Design review of the part built by this model. Coordinates are the model's own, in mm. Face numbers are marked on the shaded views. A direction names the side the tool comes from. Give positions to 0.01 mm unless a question says otherwise; leave off trailing zeros. Order: outer loops, then holes, each group sorted by start corner. A loop starts at its lowest first (then second) coordinate and runs counter-clockwise, first axis right, second up. Notation, with made-up numbers: (-24, 19) -> (27, 19) arc R23 cw to (27, 31) -> close; hole circle Ø6 at (68, -11.5). An arc over 180 degrees is marked (long way). One line per item, written item: value.
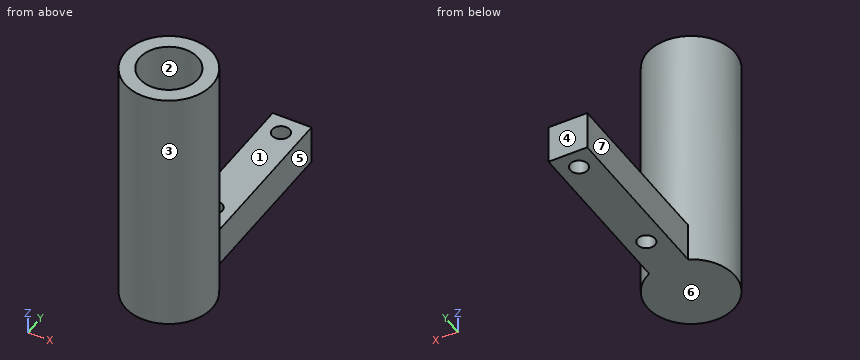
from build123d import *

# Parameters (mm, degrees)
ESQUISSE1_R             = 22.5
BASE_EXTRUSION_DEPTH    = 130
ESQUISSE2_W             = 20
ESQUISSE2_H             = 20
BOSS_EXTRU_1_DEPTH      = 110
ESQUISSE3_R             = 4.5
ENL_V_MAT_EXTRU_1_DEPTH = 20
ESQUISSE4_R             = 15
ENL_V_MAT_EXTRU_2_DEPTH = 120


with BuildPart() as part:
    # Esquisse1 → Base-Extrusion (new body)
    with BuildSketch(Plane.XY):
        with Locations(Location((0, 0, 0), (0, 0, 116.387799961))):
            Circle(ESQUISSE1_R)
    extrude(amount=BASE_EXTRUSION_DEPTH)

    # Esquisse2 → Boss.-Extru.1 (add)
    with BuildSketch(Plane(origin=(0, 0, 0), x_dir=(1, 0, 0), z_dir=(0, 1, 0))):
        with Locations((0, -10)):
            Rectangle(ESQUISSE2_W, ESQUISSE2_H)
    extrude(amount=BOSS_EXTRU_1_DEPTH)

    # Esquisse3 → Enlèv. mat.-Extru.1 (cut)
    with BuildSketch(Plane.XY.offset(20)):
        with Locations((0, 100)):
            Circle(ESQUISSE3_R)
        with Locations((0, 40)):
            Circle(ESQUISSE3_R)
    extrude(amount=-ENL_V_MAT_EXTRU_1_DEPTH, mode=Mode.SUBTRACT)

    # Esquisse4 → Enlèv. mat.-Extru.2 (cut)
    with BuildSketch(Plane.XY.offset(130)):
        Circle(ESQUISSE4_R)
    extrude(amount=-ENL_V_MAT_EXTRU_2_DEPTH, mode=Mode.SUBTRACT)


solid = part.part
Item 1: Machinability: for the marked faces 5, 6 and 7, which of the approach directions +Z, -Z, +X, -X, +Y, -Y give a long, thin tool a straight path to every point of the face, cutting with its end or side? Answer none if there is none.
Returned:
face 5: +Z, -Z, +X, +Y
face 6: -Z, +X, -X, +Y, -Y
face 7: +Z, -Z, -X, +Y
Item 2: Clearance check with flat-ended pins moving along their axes: P1, Ø10, axis at x = -17.5, z = 57.5, coming from the -Y side; P2, Ø3, axis at x = 7.5, z = 92, coming from the -Y side; P3, Ø6, axis at x = 7.5, z = 85, coming from the -Y side; P4, Ø8, axis at x = 0, y = 100, coming from the -Z side. State where each tip first meets the part, or that it passes through.
Returned:
P1: y = -18.71
P2: y = -21.69
P3: y = -22.05
P4: through
Item 3: Add section D-D on y = 0. Give the boundary of the cut face in (x, z).
Returned:
outline: (-22.5, 0) -> (22.5, 0) -> (22.5, 130) -> (15, 130) -> (15, 10) -> (-15, 10) -> (-15, 130) -> (-22.5, 130) -> close
Item 4: Add section C-C on z = 14. Give the boundary of the cut face in (x, y).
Returned:
outline: (-10, 20.16) arc R22.5 ccw (long way) to (10, 20.16) -> (10, 110) -> (-10, 110) -> close; hole circle Ø30 at (0, 0); hole circle Ø9 at (0, 40); hole circle Ø9 at (0, 100)
Item 5: To check wall thickness, follow line 1 along Y through (x, z) = (0, 13); line 2 along Y through (x, z) = (0, 9); line 3 along Y through (x, z) = (0, 69). State the ranges of each line that lie inside material, in increasing order. Write a range as from..to.
Returned:
line 1: -22.5..-15, 15..35.5, 44.5..95.5, 104.5..110
line 2: -22.5..35.5, 44.5..95.5, 104.5..110
line 3: -22.5..-15, 15..22.5
Item 6: Add section A-A on y = 100. Give the boundary of the cut face in (x, z).
Returned:
outline: (-10, 0) -> (-4.5, 0) -> (-4.5, 20) -> (-10, 20) -> close; (4.5, 0) -> (10, 0) -> (10, 20) -> (4.5, 20) -> close
Item 7: Add section B-B on x = 0.5. Give the boundary of the cut face in (y, z).
Returned:
outline: (-22.49, 0) -> (35.53, 0) -> (35.53, 20) -> (22.49, 20) -> (22.49, 130) -> (14.99, 130) -> (14.99, 10) -> (-14.99, 10) -> (-14.99, 130) -> (-22.49, 130) -> close; (44.47, 0) -> (95.53, 0) -> (95.53, 20) -> (44.47, 20) -> close; (104.47, 0) -> (110, 0) -> (110, 20) -> (104.47, 20) -> close
Item 8: Draft analysis for pull direction Y (two halves, no side actions). For the marked faces 1, 2, 3 and 4, state which applies: pulls with the +Y half, pulls with the -Y half, needs draft (parallel to the pull), parting line crosses it, or undercut.
Returned:
face 1: needs draft
face 2: undercut
face 3: parting line crosses it
face 4: pulls with the +Y half
